```python
from build123d import *

# Parameters (mm, degrees)
SCHNITT_LINEAR_AUSTRAGEN1_DEPTH = 1.5
FASE1_SIZE                      = 0.2
VERRUNDUNG1_R                   = 0.2
VERRUNDUNG2_R                   = 0.1


with BuildPart() as part:
    # Skizze1 → Rotation1 (revolve)
    with BuildSketch(Plane(origin=(0, 0, 0), x_dir=(0, 0, -1), z_dir=(1, 0, 0))):
        Polygon((-2.35, 0), (-2.35, 2.15), (0, 2.15), (0, 1.21), (25, 1.21), (25, 0), align=None)
    revolve(axis=Axis((0, 0, 21.919879518), (0, 0, -1)))

    # Skizze2 → Schnitt-Linear austragen1 (cut)
    with BuildSketch(Plane.XY.offset(2.35)):
        Polygon((1, -0.577350269), (1, 0.577350269), (0, 1.154700538), (-1, 0.577350269), (-1, -0.577350269), (0, -1.154700538), align=None)
    extrude(amount=-SCHNITT_LINEAR_AUSTRAGEN1_DEPTH, mode=Mode.SUBTRACT)

    # Fase1
    fase1_edges = [part.edges().sort_by_distance(p)[0] for p in [
        (0, -1.21, -25),
        (0, -2.15, 0),
        (0, -2.15, 2.35),
    ]]
    chamfer(fase1_edges, length=FASE1_SIZE)

    # Verrundung1
    verrundung1_edges = [part.edges().sort_by_distance(p)[0] for p in [
        (0.5, -0.866025404, 0.85),
        (1, -0.577350269, 1.6),
        (-0.5, -0.866025404, 0.85),
        (0, -1.154700538, 1.6),
        (-1, 0, 0.85),
        (-1, -0.577350269, 1.6),
        (-0.5, 0.866025404, 0.85),
        (-1, 0.577350269, 1.6),
        (0.5, 0.866025404, 0.85),
        (0, 1.154700538, 1.6),
        (1, 0, 0.85),
        (1, 0.577350269, 1.6),
        (0, -1.21, 0),
    ]]
    fillet(verrundung1_edges, radius=VERRUNDUNG1_R)

    # Verrundung2
    verrundung2_edges = [part.edges().sort_by_distance(p)[0] for p in [
        (-0.5, -0.866025404, 2.35),
        (-1, 0, 2.35),
        (-0.5, 0.866025404, 2.35),
        (0.5, 0.866025404, 2.35),
        (1, 0, 2.35),
        (0.5, -0.866025404, 2.35),
        (-0.973205081, -0.561880215, 2.35),
        (0, -1.123760431, 2.35),
        (0.973205081, -0.561880215, 2.35),
        (0.973205081, 0.561880215, 2.35),
        (0, 1.123760431, 2.35),
        (-0.973205081, 0.561880215, 2.35),
    ]]
    fillet(verrundung2_edges, radius=VERRUNDUNG2_R)


solid = part.part
```
The listing builds one solid part. Answer for the finished solid, in the listing's coordinates (mm). A direction names the side the tool comes from. Coordinates: 2 decimals unless noted, no trailing zeros. Loops run counter-clockwise (first coordinate to the right, second up) from the corner with the lowest first, then second, coordinate; pieces in that order, holes last. Notation, with made-up numbers: M -7,73.25 L 42,73.25 A22 ccw 42,100.25 Z; hole C 33,-39 d10. An arc over 180 degrees is marked long. Answer as CSV lines item,"result". Start each with the question number.
(1) Find the intervals of material crossed by L1, parallel to Z at x = -0.3, y = -0.9; L2, parallel to X at y = 0, z = -18.75; L3, parallel to Z at x = 0.1, y = -0.2, in increasing order. Write a range as [from, to].
(2) The part is cut by section A-A (y = 0). Give the vertices of the cut face in (x, z), and give its area (3 significant figures).
(3) The part is cut by section B-B (z = -6). Give the vertices of the cut face in (x, y), and give its area (3 significant figures).
(4) Given pin 1 (2 mm diameter, centred on y = -1, z = -5, fed in from +X); pin 2 (2 mm diameter, centred on y = 1, z = -2, fed in from -X); pin 3 (1 mm diameter, centred on x = 1, z = -16.5, fed in from -Y); pin 4 (2 mm diameter, centred on x = -1, y = 0.5, fed in from -Z), each flat-ended and moving along its own axis, determine where each tip first touches the part or whether it passes through.
(5) The mould has two halves that part along X. Classify faces 4 (the flat face through (0.51, 0.86, 1.66)), 5 (the cylindrical face through (0.09, -2.15, 1.16)), 6 (the flat face through (0, 0, -25)): pulls with the +X half, pulls with the -X half, needs draft (parallel to the pull), parting line crosses it, or undercut.
(6) For faces 1 (the flat face through (-0.49, 0.87, 1.66)), 2 (the flat face through (-1, -1, 2.35)), 3 (the cylindrical face through (-1.18, -0.26, -12.67)), determine the directions among +Z, -Z, +X, -X, +Y, -Y from which every point of the face is accessible in a straight line to the end or side of a thin tool.
Determined:
1,L1,"[-25, 0.9]"
1,L2,"[-1.21, 1.21]"
1,L3,"[-25, 0.85]"
2,outline,"M -2.15,0.2 L -1.95,0 L -1.41,0 A0.2 cw -1.21,-0.2 L -1.21,-24.8 L -1.01,-25 L 1.01,-25 L 1.21,-24.8 L 1.21,-0.2 A0.2 cw 1.41,0 L 1.95,0 L 2.15,0.2 L 2.15,2.15 L 1.95,2.35 L 1.1,2.35 A0.1 ccw 1,2.25 L 1,1.05 A0.2 cw 0.8,0.85 L -0.8,0.85 A0.2 cw -1,1.05 L -1,2.25 A0.1 ccw -1.1,2.35 L -1.95,2.35 L -2.15,2.15 Z"
2,area,"67.5 mm2"
3,outline,"C 0,0 d2.42"
3,area,"4.60 mm2"
4,pin 1,"x = 1.21"
4,pin 2,"x = -1.21"
4,pin 3,"y = -1.1"
4,pin 4,"z = -25"
5,face 4,"undercut"
5,face 5,"parting line crosses it"
5,face 6,"needs draft"
6,face 1,"+Z"
6,face 2,"+Z, +X, -X, +Y, -Y"
6,face 3,"-Z"
